Source: CAD feature listing. Evaluate the final solid. Frame: model axes, mm. A direction names the side the tool comes from. Coordinates: 2 decimals unless noted, no trailing zeros. Write each loop counter-clockwise with the first axis right and the second up, starting at its lowest first coordinate (ties: lowest second). Pieces come first, ordered by that corner, then holes. Notation, with made-up numbers: (40, -25.5) - (62, -25.5) arc R10 ccw to (62, -16.5) - close; hole circle Ø1 at (11.25, -13.5). An arc over 180 degrees is marked (long way). One line per question, with ' | ' between items. Start each with the question number.
Q1. Cut plane C-C, the plane y = -12.5. Return loops of the section in (x, z).
Q2. Draft query along X for faces 3 (the face through (9.5, -14, 0)), 4 (the face through (12.5, -12, 0)), 5 (the face through (-12.5, -12, 0)), 6 (the face through (-9.5, -14, 0)). Return one class per face: +X half, -X half, draft (parallel to the pull), parting line (faces both ways), or undercut.
Q3. Cut plane B-B, the plane x = 0. Return loops of the section in (y, z), plus the area to 3 significant figures.
Q4. Contact query for a flat-ended pin moving along its axis: P1, Ø10, axis at x = 0.5, z = -1.5, coming from the -Y side. Output: stop coordinate, or through.
Q5. Access query for faces 1 (the face through (0, -3, 3)), 2 (the face through (0.54, -1.48, -2.44)). Directions: +Z, -Z, +X, -X, +Y, -Y. A direction counts if a zero-diameter tool reaches every point of the face in a straight line with its end or side. Return the directions, or none.
Q6. Line query: line 1 (X direction, y = -15, z = -2.5); line 2 (Z direction, x = 0, y = -0.75); line 3 (Y direction, x = -4.75, z = 2). Output: solid intervals per line, ascending.
Q7. Cut plane D-D, the plane y = -1.75. Return loops of the section in (x, z), plus the area to 3 significant figures.
Q8. Cut plane A-A, the plane z = 0. Return loops of the section in (x, y).
```python
from build123d import *

# Parameters (mm, degrees)
F0_W     = 25
F0_H     = 25
F1_DEPTH = 25
F2_T     = -3
F4_D     = 5
F4_DEPTH = 12
F4_TIP   = 1.5021515476


with BuildPart() as f1:
    # F0 (on Front) → F1 (new body)
    with BuildSketch(Plane.XZ):
        Rectangle(F0_W, F0_H)
    extrude(amount=F1_DEPTH)

    # F2
    f2_openings = [f1.faces().sort_by_distance(p)[0] for p in [
        (0, -25, 0),
        (0, -12.5, -12.5),
        (0, -12.5, 12.5),
    ]]
    offset(amount=F2_T, openings=f2_openings)

    # F4
    with Locations(Plane.XZ.offset(3)):
        with Locations((0, 0)):
            Hole(F4_D / 2, depth=F4_DEPTH)
            with Locations((0, 0, -(F4_DEPTH + F4_TIP / 2))):  # 118° drill point
                Cone(0, F4_D / 2, F4_TIP, mode=Mode.SUBTRACT)


solid = f1.part
```
Reply:
1) outline: (-12.5, -12.5) - (-9.5, -12.5) - (-9.5, 12.5) - (-12.5, 12.5) - close; (9.5, -12.5) - (12.5, -12.5) - (12.5, 12.5) - (9.5, 12.5) - close
2) face 3: undercut | face 4: +X half | face 5: -X half | face 6: undercut
3) outline: (-3, -12.5) - (0, -12.5) - (0, -2.5) - (-3, -2.5) - close; (-3, 2.5) - (0, 2.5) - (0, 12.5) - (-3, 12.5) - close | area: 60.0 mm^2
4) P1: stops at y = -3
5) face 1: +Z, -Z, -Y | face 2: +Y, -Y
6) line 1: x = -12.5 to -9.5, 9.5 to 12.5 | line 2: z = -12.5 to -2.5, 2.5 to 12.5 | line 3: y = -3 to 0
7) outline: (-12.5, -12.5) - (12.5, -12.5) - (12.5, 12.5) - (-12.5, 12.5) - close; hole circle Ø5 at (0, 0) | area: 605 mm^2
8) outline: (-12.5, -25) - (-9.5, -25) - (-9.5, -3) - (-2.5, -3) - (-2.5, 0) - (-12.5, 0) - close; (2.5, -3) - (9.5, -3) - (9.5, -25) - (12.5, -25) - (12.5, 0) - (2.5, 0) - close
